from build123d import *

# Parameters (mm, degrees)
F0_W     = 39
F0_H     = 35
F1_DEPTH = 35
F2_W     = 33
F2_H     = 35
F3_DEPTH = 30
F4_W     = 5
F4_H     = 5
F5_DEPTH = 15
F6_W     = 5
F6_H     = 5
F7_DEPTH = 5


with BuildPart() as f1:
    # F0 (on Front) → F1 (new body)
    with BuildSketch(Plane.XZ):
        with Locations((-52.531138, 28.322564)):
            Rectangle(F0_W, F0_H)
    extrude(amount=F1_DEPTH)

    # F2 (on face) → F3 (cut)
    with BuildSketch(Plane.XZ.offset(35)):
        with Locations((-52.531138, 28.322564)):
            Rectangle(F2_W, F2_H)
    extrude(amount=-F3_DEPTH, mode=Mode.SUBTRACT)

    # F4 (on face) → F5 (join)
    with BuildSketch(Plane.YZ.offset(-33.031138)):
        with Locations((-17.5, 28.322564)):
            Rectangle(F4_W, F4_H)
    extrude(amount=F5_DEPTH)

    # F6 (on face) → F7 (join)
    with BuildSketch(Plane.YZ.offset(-18.031138)):
        with Locations((-12.5, 28.322564)):
            Rectangle(F6_W, F6_H)
    extrude(amount=-F7_DEPTH)


solid = f1.part
The listing builds one solid part. Answer for the finished solid, in the listing's coordinates (mm). A direction names the side the tool comes from. Round coordinates to 2 decimals unless told otherwise and drop trailing zeros. Write each loop counter-clockwise with the first axis right and the second up, starting at its lowest first coordinate (ties: lowest second). Pieces come first, ordered by that corner, then holes. Notation, with made-up numbers: M -15.5,46 L 27.5,46 A18 cw 27.5,55 Z; hole C 43,72 d4. An arc over 180 degrees is marked long. Write each question's results on one line, items separated by ' | '. Start each with the question number.
Item 1: For a pull along X with two mould halves and no side action, classify faces 6 (the face through (-53, -5, 29)), 7 (the face through (-18.031, -15, 28)), 8 (the face through (-72.031, -17, 28)), 9 (the face through (-24, -16, 25.823)) as pulls with the +X half, pulls with the -X half, needs draft (parallel to the pull), parting line crosses it, or undercut.
Item 2: For faces 1 (the face through (-24, -16, 30.823)), 2 (the face through (-26, -20, 28)), 3 (the face through (-69.031, -20, 28)), 4 (the face through (-20, -10, 28)), 5 (the face through (-23.031, -13, 28)), determine the directions among +Z, -Z, +X, -X, +Y, -Y from which every point of the face is accessible in a straight line to the end or side of a thin tool.
Item 3: A cutting plane is placed at A-A on y = -8. Write down the section's boundary in (x, z), and give its area (3 significant figures).
Item 4: A cutting plane is placed at B-B on y = -12.5. Write down the section's boundary in (x, z), and give its area (3 significant figures).
Item 5: A cutting plane is placed at C-C on z = 21. Write down the section's boundary in (x, y).
Item 6: A cutting plane is placed at D-D on y = -18. Write down the section's boundary in (x, z).
Item 7: Flat-ended cylindrical pins translate along their axes: pin 1 Ø2.5 at (x, z) = (-23, 29) entering from -Y; pin 2 Ø2.5 at (x, z) = (-19.5, 29.5) entering from +Y; pin 3 Ø8 at (x, y) = (-24, -14) entering from +Z. Find the tip coordinate at first contact, or state that the pin passes through.
Item 8: Straight lines are drawn through the part: L1, parallel to X at y = -20, z = 25.5; L2, parallel to Y at x = -49, z = 40; L3, parallel to X at y = -4.5, z = 33.5. For each, find the intervals that lie inside material, in ascending order. Write a range as [from, to].
Check sheet entries:
1) face 6: undercut | face 7: pulls with the +X half | face 8: pulls with the -X half | face 9: needs draft
2) face 1: +Z, +X, +Y, -Y | face 2: +Z, -Z, +X, -Y | face 3: +Z, -Z, -Y | face 4: +Z, -Z, +X, +Y | face 5: +Z, -Z, +Y
3) outline: M -72.03,10.82 L -69.03,10.82 L -69.03,45.82 L -72.03,45.82 Z; M -36.03,10.82 L -33.03,10.82 L -33.03,45.82 L -36.03,45.82 Z | area: 210 mm²
4) outline: M -72.03,10.82 L -69.03,10.82 L -69.03,45.82 L -72.03,45.82 Z; M -36.03,10.82 L -33.03,10.82 L -33.03,45.82 L -36.03,45.82 Z; M -23.03,25.82 L -18.03,25.82 L -18.03,30.82 L -23.03,30.82 Z | area: 235 mm²
5) outline: M -72.03,-35 L -69.03,-35 L -69.03,-5 L -36.03,-5 L -36.03,-35 L -33.03,-35 L -33.03,0 L -72.03,0 Z
6) outline: M -72.03,10.82 L -69.03,10.82 L -69.03,45.82 L -72.03,45.82 Z; M -36.03,10.82 L -33.03,10.82 L -33.03,25.82 L -18.03,25.82 L -18.03,30.82 L -33.03,30.82 L -33.03,45.82 L -36.03,45.82 Z
7) pin 1: y = -20 | pin 2: y = -10 | pin 3: z = 30.82
8) L1: [-72.03, -69.03], [-36.03, -33.03] | L2: [-5, 0] | L3: [-72.03, -33.03]
